from build123d import *

# Parameters (mm, degrees)
ESBO_O1_R                     = 26
ESBO_O1_R_2                   = 21
RESSALTO_EXTRUS_O1_DEPTH      = 150
CORTE_EXTRUS_O1_DEPTH         = 162.271451737
CORTE_EXTRUS_O1_DEPTH_BACK    = 162.271451737
ESBO_O3_W                     = 125
ESBO_O3_H                     = 15
RESSALTO_EXTRUS_O2_REACH      = 163.271
RESSALTO_EXTRUS_O2_END_RADIUS = 26
ESBO_O4_W                     = 15
ESBO_O4_H                     = 7
ESBO_O5_W                     = 7
ESBO_O5_H                     = 15
RESSALTO_EXTRUS_O3_DEPTH      = 10
ESBO_O6_W                     = 15
ESBO_O6_H                     = 5
RESSALTO_EXTRUS_O4_DEPTH      = 20
RESSALTO_EXTRUS_O5_REACH      = 166.697
RESSALTO_EXTRUS_O5_END_RADIUS = 26
ESBO_O7_W                     = 15
ESBO_O7_H                     = 7
ESBO_O8_W                     = 7
ESBO_O8_H                     = 15
RESSALTO_EXTRUS_O6_DEPTH      = 10
ESBO_O9_W                     = 15
ESBO_O9_H                     = 5
RESSALTO_EXTRUS_O7_DEPTH      = 20
CORTE_EXTRUS_O2_DEPTH         = 169.765720645
CORTE_EXTRUS_O2_DEPTH_BACK    = 169.765720645
ESBO_O10_R                    = 1.5
RESSALTO_EXTRUS_O8_REACH      = 165.06
RESSALTO_EXTRUS_O8_END_RADIUS = 26
ESBO_O14_W                    = 15
ESBO_O14_H                    = 20
ESBO_O15_R                    = 1.75
CORTE_EXTRUS_O3_DEPTH         = 15
CORTE_EXTRUS_O4_DEPTH         = 3
CORTE_EXTRUS_O4_DEPTH_BACK    = 18
ESBO_O17_R                    = 1.75
CORTE_EXTRUS_O5_START         = -41.1
CORTE_EXTRUS_O5_DEPTH         = 3.5
ESBO_O19_W                    = 3
ESBO_O19_H                    = 5
RESSALTO_EXTRUS_O9_DEPTH      = 5
RESSALTO_EXTRUS_O10_DEPTH     = 10
CORTE_EXTRUS_O6_DEPTH         = 163.586633287


with BuildPart() as part:
    # Esboço1 → Ressalto-extrusão1 (new body)
    with BuildSketch(Plane.XY):
        Circle(ESBO_O1_R)
        Circle(ESBO_O1_R_2, mode=Mode.SUBTRACT)
    extrude(amount=RESSALTO_EXTRUS_O1_DEPTH)

    # Esboço3 → Corte-extrusão1 (cut, two sides: drawn at the far end of the back side and taken through both)
    with BuildSketch(Plane(origin=(0, -27.221059229, 0), x_dir=(0, 0, -1), z_dir=(0, -1, 0)).offset(-CORTE_EXTRUS_O1_DEPTH_BACK)):
        with Locations((-87.5, 2.034407051)):
            Rectangle(ESBO_O3_W, ESBO_O3_H)
    extrude(amount=CORTE_EXTRUS_O1_DEPTH + CORTE_EXTRUS_O1_DEPTH_BACK, mode=Mode.SUBTRACT)

    # Ressalto-extrusão2: up to this cylinder (the profile starts outside it)
    ressalto_extrus_o2_end = Plane(origin=(0, 0, 137.5), z_dir=(0, 0, -1)) * Cylinder(RESSALTO_EXTRUS_O2_END_RADIUS, 379.542, mode=Mode.PRIVATE)
    # Esboço4 → Ressalto-extrusão2 (add, up to the surface)
    with BuildSketch(Plane(origin=(0, -27.221059229, 0), x_dir=(0, 0, -1), z_dir=(0, -1, 0)), mode=Mode.PRIVATE) as ressalto_extrus_o2_sk1:
        with Locations((-137.5, -13.965592949)):
            Rectangle(ESBO_O4_W, ESBO_O4_H)
    ressalto_extrus_o2_tool1 = extrude(ressalto_extrus_o2_sk1.sketch, amount=-RESSALTO_EXTRUS_O2_REACH, mode=Mode.PRIVATE) - ressalto_extrus_o2_end
    add(ressalto_extrus_o2_tool1.solids().sort_by_distance((-13.965593, -27.221059, 137.5))[0])

    # Esboço5 → Ressalto-extrusão3 (add)
    with BuildSketch(Plane.XZ.offset(27.221059229)):
        with Locations((-13.965592949, 137.5)):
            Rectangle(ESBO_O5_W, ESBO_O5_H)
    extrude(amount=RESSALTO_EXTRUS_O3_DEPTH)

    # Esboço6 → Ressalto-extrusão4 (add)
    with BuildSketch(Plane(origin=(-10.465592949, 0, 0), x_dir=(0, 0, -1), z_dir=(1, 0, 0))):
        with Locations((-137.5, -34.721059229)):
            Rectangle(ESBO_O6_W, ESBO_O6_H)
    extrude(amount=RESSALTO_EXTRUS_O4_DEPTH)

    # Ressalto-extrusão5: up to this cylinder (the profile starts outside it)
    ressalto_extrus_o5_end = Plane(origin=(0, 0, 137.5), z_dir=(0, 0, -1)) * Cylinder(RESSALTO_EXTRUS_O5_END_RADIUS, 386.394, mode=Mode.PRIVATE)
    # Esboço7 → Ressalto-extrusão5 (add, up to the surface)
    with BuildSketch(Plane.ZX.offset(25.620333295), mode=Mode.PRIVATE) as ressalto_extrus_o5_sk1:
        with Locations((137.5, -13.965592949)):
            Rectangle(ESBO_O7_W, ESBO_O7_H)
    ressalto_extrus_o5_tool1 = extrude(ressalto_extrus_o5_sk1.sketch, amount=-RESSALTO_EXTRUS_O5_REACH, mode=Mode.PRIVATE) - ressalto_extrus_o5_end
    add(ressalto_extrus_o5_tool1.solids().sort_by_distance((-13.965593, 25.620333, 137.5))[0])

    # Esboço8 → Ressalto-extrusão6 (add)
    with BuildSketch(Plane(origin=(0, 25.620333295, 0), x_dir=(1, 0, 0), z_dir=(0, 1, 0))):
        with Locations((-13.965592949, -137.5)):
            Rectangle(ESBO_O8_W, ESBO_O8_H)
    extrude(amount=RESSALTO_EXTRUS_O6_DEPTH)

    # Esboço9 → Ressalto-extrusão7 (add)
    with BuildSketch(Plane(origin=(-10.465592949, 0, 0), x_dir=(0, 0, -1), z_dir=(1, 0, 0))):
        with Locations((-137.5, 33.120333295)):
            Rectangle(ESBO_O9_W, ESBO_O9_H)
    extrude(amount=RESSALTO_EXTRUS_O7_DEPTH)

    # Esboço10 → Corte-extrusão2 (cut, two sides: drawn at the far end of the back side and taken through both)
    with BuildSketch(Plane.XZ.offset(37.221059229).offset(-CORTE_EXTRUS_O2_DEPTH_BACK)):
        with Locations((-13.4052452, 137.5)):
            Circle(ESBO_O10_R)
    extrude(amount=CORTE_EXTRUS_O2_DEPTH + CORTE_EXTRUS_O2_DEPTH_BACK, mode=Mode.SUBTRACT)

    # Ressalto-extrusão8: up to this cylinder (the profile starts outside it)
    ressalto_extrus_o8_end = Plane(origin=(0, 0, 65), z_dir=(0, 0, -1)) * Cylinder(RESSALTO_EXTRUS_O8_END_RADIUS, 458.562278, mode=Mode.PRIVATE)
    # Esboço14 → Ressalto-extrusão8 (add, up to the surface)
    with BuildSketch(Plane(origin=(-25.991571687, 0, 0), x_dir=(0, -1, 0), z_dir=(-1, 0, 0)), mode=Mode.PRIVATE) as ressalto_extrus_o8_sk1:
        with Locations((-11.76014182, 102.721139131)):
            Rectangle(ESBO_O14_W, ESBO_O14_H)
    ressalto_extrus_o8_tool1 = extrude(ressalto_extrus_o8_sk1.sketch, amount=-RESSALTO_EXTRUS_O8_REACH, mode=Mode.PRIVATE) - ressalto_extrus_o8_end
    add(ressalto_extrus_o8_tool1.solids().sort_by_distance((-25.991572, 11.760142, 102.721139))[0])
    # Esboço14 → Ressalto-extrusão8 (add, up to the surface)
    with BuildSketch(Plane(origin=(-25.991571687, 0, 0), x_dir=(0, -1, 0), z_dir=(-1, 0, 0)), mode=Mode.PRIVATE) as ressalto_extrus_o8_sk2:
        with Locations((11.76014182, 102.721139131)):
            Rectangle(ESBO_O14_W, ESBO_O14_H)
    ressalto_extrus_o8_tool2 = extrude(ressalto_extrus_o8_sk2.sketch, amount=-RESSALTO_EXTRUS_O8_REACH, mode=Mode.PRIVATE) - ressalto_extrus_o8_end
    add(ressalto_extrus_o8_tool2.solids().sort_by_distance((-25.991572, -11.760142, 102.721139))[0])
    # Esboço14 → Ressalto-extrusão8 (add, up to the surface)
    with BuildSketch(Plane(origin=(-25.991571687, 0, 0), x_dir=(0, -1, 0), z_dir=(-1, 0, 0)), mode=Mode.PRIVATE) as ressalto_extrus_o8_sk3:
        with Locations((11.76014182, 27.278860869)):
            Rectangle(ESBO_O14_W, ESBO_O14_H)
    ressalto_extrus_o8_tool3 = extrude(ressalto_extrus_o8_sk3.sketch, amount=-RESSALTO_EXTRUS_O8_REACH, mode=Mode.PRIVATE) - ressalto_extrus_o8_end
    add(ressalto_extrus_o8_tool3.solids().sort_by_distance((-25.991572, -11.760142, 27.278861))[0])
    # Esboço14 → Ressalto-extrusão8 (add, up to the surface)
    with BuildSketch(Plane(origin=(-25.991571687, 0, 0), x_dir=(0, -1, 0), z_dir=(-1, 0, 0)), mode=Mode.PRIVATE) as ressalto_extrus_o8_sk4:
        with Locations((-11.76014182, 27.278860869)):
            Rectangle(ESBO_O14_W, ESBO_O14_H)
    ressalto_extrus_o8_tool4 = extrude(ressalto_extrus_o8_sk4.sketch, amount=-RESSALTO_EXTRUS_O8_REACH, mode=Mode.PRIVATE) - ressalto_extrus_o8_end
    add(ressalto_extrus_o8_tool4.solids().sort_by_distance((-25.991572, 11.760142, 27.278861))[0])

    # Esboço15 → Corte-extrusão3 (cut)
    with BuildSketch(Plane.ZY.offset(25.991571687)):
        with Locations((27.278860869, 11.76014182)):
            Circle(ESBO_O15_R)
        with Locations((102.721139131, 11.76014182)):
            Circle(ESBO_O15_R)
        with Locations((102.721139131, -11.76014182)):
            Circle(ESBO_O15_R)
        with Locations((27.278860869, -11.76014182)):
            Circle(ESBO_O15_R)
    extrude(amount=-CORTE_EXTRUS_O3_DEPTH, mode=Mode.SUBTRACT)

    # Esboço17 → Corte-extrusão4 (cut, two sides: drawn at the far end of the back side and taken through both)
    with BuildSketch(Plane(origin=(0, -27.221059229, 0), x_dir=(0, 0, -1), z_dir=(0, -1, 0)).offset(-CORTE_EXTRUS_O4_DEPTH_BACK)):
        with Locations(Location((-19, 2.034407051, 0), (0, 0, 90))):
            Circle(ESBO_O17_R)
        with Locations(Location((-6, 2.034407051, 0), (0, 0, 90))):
            Circle(ESBO_O17_R)
    extrude(amount=CORTE_EXTRUS_O4_DEPTH + CORTE_EXTRUS_O4_DEPTH_BACK, mode=Mode.SUBTRACT)

    # Esboço18 → Corte-extrusão5 (cut)
    with BuildSketch(Plane.ZX.offset(20.835810462).offset(CORTE_EXTRUS_O5_START)):
        Polygon((9, 0.302356243), (9, 3.766457858), (6, 5.498508666), (3, 3.766457858), (3, 0.302356243), (6, -1.429694564), align=None)
        Polygon((21.989029976, 3.785321041), (18.978178993, 5.498439938), (15.989149016, 3.747525948), (16.010970024, 0.283493061), (19.021821007, -1.429625836), (22.010850984, 0.321288154), align=None)
    extrude(amount=-CORTE_EXTRUS_O5_DEPTH, mode=Mode.SUBTRACT)

    # Esboço19 → Ressalto-extrusão9 (add)
    with BuildSketch(Plane.XY.offset(150)):
        with Locations((-23.057246572, 2.5)):
            Rectangle(ESBO_O19_W, ESBO_O19_H)
        with Locations((-23.057246572, -2.5)):
            Rectangle(ESBO_O19_W, ESBO_O19_H)
    extrude(amount=RESSALTO_EXTRUS_O9_DEPTH)

    # Esboço20 → Ressalto-extrusão10 (add)
    with BuildSketch(Plane(origin=(0, 5, 0), x_dir=(1, 0, 0), z_dir=(0, 1, 0))):
        Polygon((-24.557246572, -155), (-24.557246572, -152), (-27.557246572, -155), align=None)
    extrude(amount=-RESSALTO_EXTRUS_O10_DEPTH)

    # Esboço23 → Corte-extrusão6 (cut, through all)
    with BuildSketch(Plane.XZ.offset(5)):
        Polygon((-27.557246572, 155), (-25.991571687, 155), (-26.057246572, 153.5), align=None)
    extrude(amount=-CORTE_EXTRUS_O6_DEPTH, mode=Mode.SUBTRACT)


solid = part.part
Build history of the part. All positions in model axes, mm. A direction names the side the tool comes from. Give positions to 0.01 mm unless a question says otherwise; leave off trailing zeros. Order: outer loops, then holes, each group sorted by start corner. A loop starts at its lowest first (then second) coordinate and runs counter-clockwise, first axis right, second up. Notation, with made-up numbers: M -38.75,32.25 L -11.75,32.25 A18 ccw -11.75,40.25 Z; hole C -25.5,1 d1. An arc over 180 degrees is marked long. Put each result on its own line as item: value.
Item 1: 3-axis set-ups, long thin cutter, end or side, ignore diameter. For faces 1 (the cylindrical face through (-22.2, 13.5, 27.1)), 2 (the flat face through (2, -23, 25)), 3 (the flat face through (-22, -19.26, 103)), 4 (the flat face through (-23, 5, 152)): which of +Z, -Z, +X, -X, +Y, -Y reach the whole face in a straight line?
From the geometry:
face 1: -X
face 2: +Z, +Y, -Y
face 3: +Z, -Z, -X, -Y
face 4: +Z, +X, -X, +Y
Item 2: Slice it at D-D, the plane z = 137.5. Write the cut outline in (x, y).
From the geometry:
outline: M -17.47,-37.22 L -14.91,-37.22 L -14.91,-14.79 A21 cw -14.91,14.79 L -14.91,35.62 L -17.47,35.62 L -17.47,19.26 A26 ccw -17.47,-19.26 Z; M -11.91,-37.22 L 9.53,-37.22 L 9.53,-32.22 L -10.47,-32.22 L -10.47,-23.8 A26 ccw -5.47,-25.42 L -5.47,-20.28 A21 cw -11.91,-17.3 Z; M -11.91,17.3 A21 cw -5.47,20.28 L -5.47,25.42 A26 ccw -10.47,23.8 L -10.47,30.62 L 9.53,30.62 L 9.53,35.62 L -11.91,35.62 Z; M 9.53,-24.19 A26 ccw 9.53,24.19 L 9.53,18.71 A21 cw 9.53,-18.71 Z
Item 3: Slice it at C-C, the plane y = 28.5. Write the cut outline in (x, z), plus the area to 3 significant figures.
From the geometry:
outline: M -17.47,130 L -10.47,130 L -10.47,145 L -17.47,145 Z; hole C -13.41,137.5 d3
area: 97.9 mm2
Item 4: Two-plate mould, pull along Y, no slides. Class faces 5 (the flat face through (-25.992, 14, 103)), 6 (the flat face through (-4, 35.62, 138)), 7 (the flat face through (-10.466, -28, 137)): +Y half, -Y half, draft (parallel to the pull), parting line (faces both ways), or undercut.
From the geometry:
face 5: draft
face 6: +Y half
face 7: undercut
Item 5: Flat gauge pins, fed straight in: pin 1 Ø2.5 at (x, z) = (-23, 23) entering from -Y; pin 2 Ø6 at (y, z) = (-16.5, 93.5) entering from -X; pin 3 Ø10 at (y, z) = (-28.5, 138) entering from +X. Where does each tip first touch, or does it go through?
From the geometry:
pin 1: stops at y = -19.26
pin 2: stops at x = -25.99
pin 3: stops at x = 11.12
Item 6: Probe line 1 (Z direction, x = -23, y = 12); line 2 (Y direction, x = -7.5, z = 135); line 3 (X direction, y = -21, z = 137). List the from-to ranges inside material, lowest first. Write a range as [from, to].
From the geometry:
line 1: z = [0, 25.55], [29.01, 100.99], [104.45, 150]
line 2: y = [-37.22, -32.22], [-24.89, -19.62], [19.62, 24.89], [30.62, 35.62]
line 3: x = [-17.47, -14.82], [-11.99, -5.47], [9.53, 15.33]
Item 7: Slice it at B-B, the plane x = -19.5. Write the cut outline in (y, z).
From the geometry:
outline: M -19.26,17.28 L -17.2,17.28 L -17.2,0 L -7.79,0 L -7.79,150 L -17.2,150 L -17.2,112.72 L -19.26,112.72 L -19.26,92.72 L -17.2,92.72 L -17.2,37.28 L -19.26,37.28 Z; M 7.79,0 L 17.2,0 L 17.2,17.28 L 19.26,17.28 L 19.26,37.28 L 17.2,37.28 L 17.2,92.72 L 19.26,92.72 L 19.26,112.72 L 17.2,112.72 L 17.2,150 L 7.79,150 Z; hole C -11.76,27.28 d3.5; hole C -11.76,102.72 d3.5; hole C 11.76,27.28 d3.5; hole C 11.76,102.72 d3.5
Item 8: Slice it at A-A, the plane z = 58. Write the cut outline in (x, y).
From the geometry:
outline: M -5.47,-25.42 L -5.47,-20.28 A21 cw -5.47,20.28 L -5.47,25.42 A26 ccw Z; M 9.53,-24.19 A26 ccw 9.53,24.19 L 9.53,18.71 A21 cw 9.53,-18.71 Z
